Autodesk Inventor part; units mm, degrees
ref_plane "YZ Plane" through (0, 0, 0) normal (1, 0, 0) x (0, 1, 0)
ref_plane "XZ Plane" through (0, 0, 0) normal (0, 1, 0) x (-1, 0, 0)
ref_plane "XY Plane" through (0, 0, 0) normal (0, 0, 1) x (1, 0, 0)
sketch "スケッチ1" plane through (0, 0, 0) normal (0, 1, 0) x (-1, 0, 0)
  line L0 (25, 0) -> (-25, 0)
  line L1 (-25, 0) -> (-25, -159)
  line L2 (-25, -159) -> (25, -159)
  line L3 (25, -159) -> (25, 0)
  circle A0 centre (0, 0) radius 25
  circle A1 centre (0, 0) radius 57 construction
  circle A2 centre (0, -79.5) radius 22.5 construction
  circle A3 centre (0, 0) radius 75 construction
  circle A4 centre (0, -79.5) radius 10
  circle A5 centre (0, 0) radius 10
  circle A6 centre (0, -159) radius 10
  circle A7 centre (0, -159) radius 57 construction
  circle A8 centre (0, -159) radius 25
  dimension "d0" = 114
  dimension "d1" = 45
  dimension "d2" = 150
  dimension "d3" = 20
  dimension "d4" = 20
  dimension "d5" = 50
  dimension "d8" = 20
extrude "押し出し1" add sketch "スケッチ1" along normal blind 5 contours A0 L0 A5 | L0 A5 A0 | L3 A8 L1 A0 | A8 L2 A6 | L2 A6 A8
sketch "スケッチ2" plane through (0, 0, 0) normal (0, -1, 0) x (1, 0, 0)
  line L0 (60, -134) -> (-60, -134)
  line L1 (-60, -134) -> (-60, -184)
  line L2 (-60, -184) -> (60, -184)
  line L3 (60, -184) -> (60, -134)
  line L4 (25, 0) -> (25, -159)
  arc A0 (25, 0) -> (-25, 0) centre (0, 0) ccw
  line L5 (-25, -159) -> (-25, 0)
  arc A1 (-25, -159) -> (25, -159) centre (0, -159) ccw
  circle A2 centre (0, 0) radius 10
  circle A3 centre (0, -79.5) radius 10
  circle A4 centre (0, -159) radius 10
  arc A5 (-25, -159) -> (25, -159) centre (0, -159) ccw
  point P0 (0, -184)
  point P1 (25, -134)
  point P2 (0, -184)
  point P3 (-25, -134)
  dimension "d9" = 120
  dimension "d10" = 50
extrude "押し出し2" add sketch "スケッチ2" against normal up to surface (5 mm away) contours L3 L2 A1 L4 L0 | L5 A1 L2 L1 L0
sketch "スケッチ3" plane through (0, 5, 0) normal (0, 1, 0) x (1, 0, 0)
  line L0 (-60, 184) -> (60, 184)
  line L1 (-25, 134) -> (25, 134)
  line L2 (25, 134) -> (25, 184)
  line L3 (25, 184) -> (-25, 184)
  line L4 (-25, 184) -> (-25, 134)
  line L5 (-25, 184) -> (-30.5, 184)
  line L6 (-30.5, 184) -> (-30.5, 174)
  line L7 (-30.5, 174) -> (-25, 174)
  line L8 (-25, 174) -> (-25, 184)
  line L9 (25, 184) -> (30.5, 184)
  line L10 (30.5, 184) -> (30.5, 174)
  line L11 (30.5, 174) -> (25, 174)
  line L12 (25, 174) -> (25, 184)
  line L13 (-25, 134) -> (-60, 134)
  line L14 (-25, 134) -> (-30.5, 134)
  line L15 (-30.5, 134) -> (-30.5, 144)
  line L16 (-30.5, 144) -> (-25, 144)
  line L17 (-25, 144) -> (-25, 134)
  line L18 (25, 134) -> (30.5, 134)
  line L19 (30.5, 134) -> (30.5, 144)
  line L20 (30.5, 144) -> (25, 144)
  line L21 (25, 144) -> (25, 134)
  point P0 (0, 0)
  point P1 (25, 174)
  point P2 (-25, 144)
  point P3 (-25, 174)
  point P4 (-25, 184)
  dimension "d13" = 5.5
  dimension "d14" = 5.5
  dimension "d15" = 10
extrude "押し出し3" cut sketch "スケッチ3" against normal through all contours L0 L4 L7 L6 | L0 L10 L11 L2 | L4 L13 L15 L16 | L20 L19 L18 L2
equation "\"d14\" = d13"
properties part number "ギアプレート"
Read the model definition and answer for the solid it produces. Units are mm, in the model's axes. A direction names the side the tool comes from. Coordinates: 2 decimals unless noted, no trailing zeros. Order: outer loops, then holes, each group sorted by start corner. A loop starts at its lowest first (then second) coordinate and runs counter-clockwise, first axis right, second up. Notation, with made-up numbers: (35, 70) - (50, 70) arc R25 ccw to (50, 108) - close; hole circle Ø1 at (83, -1.5). An arc over 180 degrees is marked (long way). Use one line per item in the form item = value.
(1) Section C-C, the plane z = -137 is taken. Give the vertices of the cut face in (x, y), then the cut area to 3 significant figures.
Computed values:
outline = (-60, 0) - (-30.5, 0) - (-30.5, 5) - (-60, 5) - close; (-25, 0) - (25, 0) - (25, 5) - (-25, 5) - close; (30.5, 0) - (60, 0) - (60, 5) - (30.5, 5) - close
area = 545 mm²
(2) For a pull along X with two mould halves and no side action, classify faces 6 (the face through (-60, 2, -159)), 7 (the face through (0, 2, -184)), 8 (the face through (25, 3, -179)) as pulls with the +X half, pulls with the -X half, needs draft (parallel to the pull), parting line crosses it, or undercut.
Computed values:
face_6 = pulls with the -X half
face_7 = needs draft
face_8 = undercut
(3) Section A-A, the plane x = 0 is taken. Give the vertices of the cut face in (y, z), then the cut area to 3 significant figures.
Computed values:
outline = (0, -184) - (5, -184) - (5, -169) - (0, -169) - close; (0, -149) - (5, -149) - (5, -89.5) - (0, -89.5) - close; (0, -69.5) - (5, -69.5) - (5, -10) - (0, -10) - close; (0, 10) - (5, 10) - (5, 25) - (0, 25) - close
area = 745 mm²
(4) Straight lines are drawn through the part: L1, parallel to Z at x = 0, y = 2.4; L2, parallel to X at y = 3.25, z = 0; L3, parallel to Z at x = 7, y = 2.2. For each, find the intervals that lie inside material, in ascending order.
Computed values:
L1 = -184 to -169, -149 to -89.5, -69.5 to -10, 10 to 25
L2 = -25 to -10, 10 to 25
L3 = -184 to -166.14, -151.86 to -86.64, -72.36 to -7.14, 7.14 to 24
(5) Which of the six approach directions +Z, -Z, +X, -X, +Y, -Y give full straight-line access (tool end or side, diameter ignored) to faces 1 (the face through (45, 2, -134)), 2 (the face through (1.302, 2.465, -89.415)), 3 (the face through (-28, 3, -144)), 4 (the face through (-28, 3, -174)), 5 (the face through (-45, 2, -134))?
Computed values:
face_1 = +Z, +X, +Y, -Y
face_2 = +Y, -Y
face_3 = +Z, +Y, -Y
face_4 = -Z, +Y, -Y
face_5 = +Z, -X, +Y, -Y
(6) Section D-D, the plane y = 1.1 is taken. Give the vertices of the cut face in (x, z), then the cut area to 3 significant figures.
Computed values:
outline = (-60, -184) - (-30.5, -184) - (-30.5, -174) - (-25, -174) - (-25, -184) - (25, -184) - (25, -174) - (30.5, -174) - (30.5, -184) - (60, -184) - (60, -134) - (30.5, -134) - (30.5, -144) - (25, -144) - (25, 0) arc R25 ccw to (-25, 0) - (-25, -144) - (-30.5, -144) - (-30.5, -134) - (-60, -134) - close; hole circle Ø20 at (0, -159); hole circle Ø20 at (0, -79.5); hole circle Ø20 at (0, 0)
area = 12,500 mm²
(7) Given pin 1 Ø2.5 at (x, y) = (43.5, 3) entering from +Z; pin 2 Ø6 at (x, z) = (2.5, -56) entering from -Y; pin 3 Ø2 at (y, z) = (2.5, -71) entering from +X; pin 4 Ø2.5 at (x, y) = (28.5, 1.5) entering from -Z, each flat-ended and moving along its own axis, determine where each tip first touches the part or whether it passes through.
Computed values:
pin_1 = -134
pin_2 = 0
pin_3 = 25
pin_4 = -174
(8) Section B-B, the plane z = -159 is taken. Give the vertices of the cut face in (x, y), then the cut area to 3 significant figures.
Computed values:
outline = (-60, 0) - (-10, 0) - (-10, 5) - (-60, 5) - close; (10, 0) - (60, 0) - (60, 5) - (10, 5) - close
area = 500 mm²
